For this review, take the finished solid that the model builds, in its own axes (mm). Face numbers are marked on the shaded views. A direction names the side the tool comes from. Give positions to 0.01 mm unless a question says otherwise; leave off trailing zeros. Order: outer loops, then holes, each group sorted by start corner. A loop starts at its lowest first (then second) coordinate and runs counter-clockwise, first axis right, second up. Notation, with made-up numbers: (65, 13) - (83, 13) arc R18 ccw to (83, 23) - close; hole circle Ø1 at (89, 75). An arc over 180 degrees is marked (long way). One line per item, written item: value.
Autodesk Inventor part; units mm, degrees
ref_plane "YZ Plane" through (0, 0, 0) normal (1, 0, 0) x (0, 1, 0)
ref_plane "XZ Plane" through (0, 0, 0) normal (0, 1, 0) x (-1, 0, 0)
ref_plane "XY Plane" through (0, 0, 0) normal (0, 0, 1) x (1, 0, 0)
sketch "스케치1" plane through (0, 0, 0) normal (0, 1, 0) x (-1, 0, 0)
  circle A0 centre (0, 0) radius 1.6
  circle A1 centre (0, 0) radius 2.4
  circle A2 centre (0, -4.8) radius 2.4
  circle A3 centre (0, -4.8) radius 1.6
  line L0 (1.6, 0) -> (1.6, -4.8)
  line L1 (-1.6, 0) -> (-1.6, -4.8)
  line L2 (-2.4, 2.4) -> (2.4, 2.4)
  line L3 (2.4, 2.4) -> (2.4, -7.2)
  line L4 (2.4, -7.2) -> (-2.4, -7.2)
  line L5 (-2.4, -7.2) -> (-2.4, 2.4)
  point P0 (0, -2.4)
  dimension "d1" = 4.8
  dimension "d2" = 4.8
  dimension "d0" = 3.2
  dimension "d3" = 3.2
extrude "돌출3" add sketch "스케치1" against normal blind 2 contours L0 A1 L1 A0 | A0 L1 A1 L0 | L0 A2 A1 | A1 L3 A2 L0 | L1 A2 L5 A1 | A1 A2 L1 | A2 L0 A3 L1 | A1 L2 L3 | A2 L1 A3 L0 | L5 L2 A1 | L3 L4 A2 | A2 L4 L5
extrude "돌출4" add sketch "스케치1" along normal blind 4 contours A0 L1 A1 L0 | A1 L3 A2 L0 | L1 A2 L5 A1 | A1 L2 L3 | A2 L1 A3 L0 | L5 L2 A1 | L3 L4 A2 | A2 L4 L5 picked at (-1.7127, -1.0681) picked at (-1.7127, -3.7319)
sketch "스케치2" plane through (0, 4, 0) normal (0, 1, 0) x (1, 0, 0)
  line L0 (-2.4, -2.4) -> (2.4, -2.4)
  line L1 (2.4, -2.4) -> (2.4, 7.2)
  line L2 (2.4, 7.2) -> (-2.4, 7.2)
  line L3 (-2.4, 7.2) -> (-2.4, -2.4)
  line L4 (-1.6, 0) -> (-1.6, 4.8)
  arc A0 (1.6, 4.8) -> (-1.6, 4.8) centre (0, 4.8) ccw
  line L5 (1.6, 4.8) -> (1.6, 0)
  arc A1 (-1.6, 0) -> (1.6, 0) centre (0, 0) ccw
extrude "돌출5" add sketch "스케치2" against normal blind 0.8 contours L3 L2 L1 L0 | L4 A0 L5 A1
sketch "스케치3" plane through (2.4, -2, -7.2) normal (0, 0, -1) x (-1, 0, 0)
  circle A0 centre (2.4, 3.6) radius 1.6
  line L0 (0, 6) -> (4.8, 6)
  circle A1 centre (2.4, 3.6) radius 2.4
  line L1 (4.8, 0) -> (4.8, 6)
  point P0 (2.4, 2)
  dimension "d14" = 3.2
  dimension "d15" = 2.4
  dimension "d16" = 4.8
extrude "돌출6" cut sketch "스케치3" against normal blind 3.3 contours A0
properties part number "endcap_4mm_2ea_typeB_ver2_onyx"
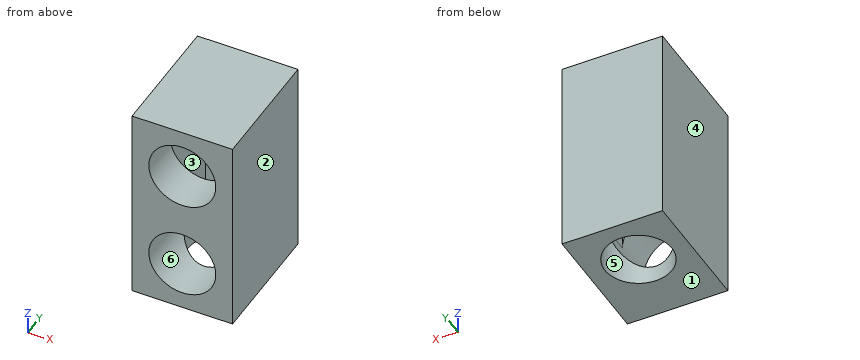
(1) Take a section at B-B (y = -0.15). Write out the cut boundary in (x, z), then the cut area to 3 significant figures.
Answers below:
outline: (-2.4, -7.2) - (2.4, -7.2) - (2.4, 2.4) - (-2.4, 2.4) - close; hole circle Ø3.2 at (0, -4.8); hole circle Ø3.2 at (0, 0)
area: 30.0 mm^2
(2) Take a section at D-D (y = 1.75). Write out the cut boundary in (x, z).
Answers below:
outline: (-2.4, -7.2) - (-1.59, -7.2) - (-1.59, -4.95) arc R1.6 cw to (-1.6, -4.8) - (-1.6, 0) arc R1.6 cw to (1.6, 0) - (1.6, -4.8) arc R1.6 cw to (1.59, -4.95) - (1.59, -7.2) - (2.4, -7.2) - (2.4, 2.4) - (-2.4, 2.4) - close
(3) Wall thickness on line 1 (Z direction, x = 0, y = -0.7); line 2 (Y direction, x = -0.8, z = -2.5); line 3 (X direction, y = 3.05, z = -4): over which ranges is each line inside the solid? List them lowest first. Write a range as from..to.
Answers below:
line 1: z = -7.2..-6.4, -3.2..-1.6, 1.6..2.4
line 2: y = -2..0, 3.2..4
line 3: x = -2.4..-1.6, 1.6..2.4
(4) Take a section at A-A (x = 1.3). Write out the cut boundary in (y, z).
Answers below:
outline: (-2, -7.2) - (0.67, -7.2) - (0.67, -5.73) - (-2, -5.73) - close; (-2, -3.87) - (0, -3.87) - (0, -0.93) - (-2, -0.93) - close; (-2, 0.93) - (3.2, 0.93) - (3.2, -5.73) - (2.53, -5.73) - (2.53, -7.2) - (4, -7.2) - (4, 2.4) - (-2, 2.4) - close
(5) Take a section at C-C (z = -5.5). Write out the cut boundary in (x, y).
Answers below:
outline: (-2.4, -2) - (-1.44, -2) - (-1.44, 0.9) arc R1.6 cw to (-1.44, 2.3) - (-1.44, 3.2) - (1.44, 3.2) - (1.44, 2.3) arc R1.6 cw to (1.44, 0.9) - (1.44, -2) - (2.4, -2) - (2.4, 4) - (-2.4, 4) - close
(6) Machinability: for the marked faces 4, 5 and 6, which of the approach directions +Z, -Z, +X, -X, +Y, -Y give a long, thin tool a straight path to every point of the face, cutting with its end or side? Answer none if there is none.
Answers below:
face 4: +Z, -Z, -X, +Y, -Y
face 5: -Z
face 6: -Y
(7) Draft analysis for pull direction Z (two halves, no side actions). For the marked faces 1, 2 and 3, state which applies: pulls with the +Z half, pulls with the -Z half, needs draft (parallel to the pull), parting line crosses it, or undercut.
Answers below:
face 1: pulls with the -Z half
face 2: needs draft
face 3: undercut
